Input: part model. Units: mm. Frame: model coordinates. Face numbers are marked on the shaded views. A direction names the side the tool comes from. Give positions to 0.01 mm unless a question says otherwise; leave off trailing zeros. Write each loop counter-clockwise with the first axis right and the second up, starting at its lowest first coordinate (ties: lowest second). Pieces come first, ordered by that corner, then holes. Notation, with made-up numbers: M -34,-40 L -14,-40 A15 cw -14,-27 Z; hole C 12.25,34.25 d7. An arc over 180 degrees is marked long. Use CSV: the item, a comma, the result in double quotes. Start each with the question number.
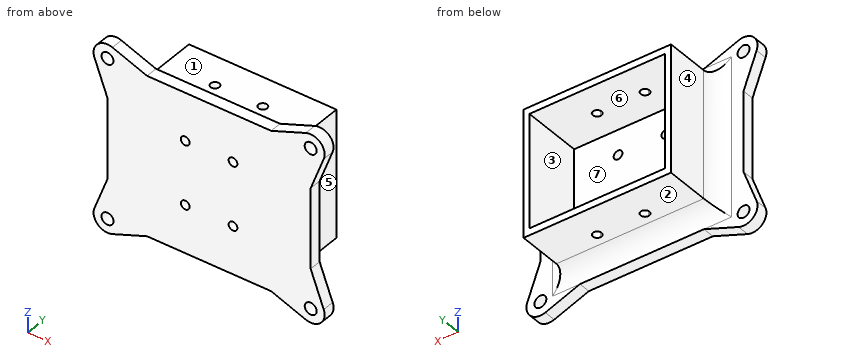
from build123d import *

# Parameters (mm, degrees)
SKETCH1_R               = 1.5
BOSS_EXTRUDE2_DEPTH     = 3
SKETCH2_W               = 37
SKETCH2_H               = 32
SKETCH2_W_2             = 34.05
SKETCH2_H_2             = 28.55
BOSS_EXTRUDE3_DEPTH     = 15
CUT_EXTRUDE1_DEPTH      = 40
CUT_EXTRUDE1_DEPTH_BACK = 11
SKETCH2_4_R             = 1.1
CUT_EXTRUDE2_DEPTH      = 11
FILLET1_R               = 4


with BuildPart() as part:
    # Sketch1 → Boss-Extrude2 (new body)
    with BuildSketch(Plane(origin=(0, 0, 0), x_dir=(1, 0, 0), z_dir=(0, 1, 0))):
        with BuildLine():
            Line((-24.266499455, 23.2754353), (-15.568913997, 20))
            Line((-15.568913997, 20), (15.568913997, 20))
            Line((15.568913997, 20), (24.266499455, 23.2754353))
            ThreePointArc((24.266499455, 23.2754353), (27.974873734, 22.474873734), (28.7754353, 18.766499455))
            Line((28.7754353, 18.766499455), (25.5, 10.068913997))
            Line((25.5, 10.068913997), (25.5, -10.068913997))
            Line((25.5, -10.068913997), (28.7754353, -18.766499455))
            ThreePointArc((28.7754353, -18.766499455), (27.974873734, -22.474873734), (24.266499455, -23.2754353))
            Line((24.266499455, -23.2754353), (15.568913997, -20))
            Line((15.568913997, -20), (-15.568913997, -20))
            Line((-15.568913997, -20), (-24.266499455, -23.2754353))
            ThreePointArc((-24.266499455, -23.2754353), (-27.974873734, -22.474873734), (-28.7754353, -18.766499455))
            Line((-28.7754353, -18.766499455), (-25.5, -10.068913997))
            Line((-25.5, -10.068913997), (-25.5, 10.068913997))
            Line((-25.5, 10.068913997), (-28.7754353, 18.766499455))
            ThreePointArc((-28.7754353, 18.766499455), (-27.974873734, 22.474873734), (-24.266499455, 23.2754353))
        make_face()
        with Locations(Location((-25.5, 20, 0), (0, 0, 270))):
            Circle(SKETCH1_R, mode=Mode.SUBTRACT)
        with Locations(Location((25.5, 20, 0), (0, 0, 270))):
            Circle(SKETCH1_R, mode=Mode.SUBTRACT)
        with Locations(Location((25.5, -20, 0), (0, 0, 270))):
            Circle(SKETCH1_R, mode=Mode.SUBTRACT)
        with Locations(Location((-25.5, -20, 0), (0, 0, 270))):
            Circle(SKETCH1_R, mode=Mode.SUBTRACT)
    extrude(amount=BOSS_EXTRUDE2_DEPTH)

    # Sketch2 → Boss-Extrude3 (add)
    with BuildSketch(Plane(origin=(0, 3, 0), x_dir=(1, 0, 0), z_dir=(0, 1, 0))):
        Rectangle(SKETCH2_W, SKETCH2_H)
        Rectangle(SKETCH2_W_2, SKETCH2_H_2, mode=Mode.SUBTRACT)
    extrude(amount=BOSS_EXTRUDE3_DEPTH)

    # Sketch3 → Cut-Extrude1 (cut, two sides: drawn at the far end of the back side and taken through both)
    with BuildSketch(Plane.XY.offset(-14.275).offset(-CUT_EXTRUDE1_DEPTH_BACK)):
        with BuildLine():
            ThreePointArc((-4.9, 10), (-6.777817459, 10.777817459), (-6, 8.9))
            Line((-6, 8.9), (-6, 10))
            Line((-6, 10), (-4.9, 10))
        make_face()
        with BuildLine():
            Line((-6, 10), (-6, 8.9))
            ThreePointArc((-6, 8.9), (-5.222182541, 9.222182541), (-4.9, 10))
            Line((-4.9, 10), (-6, 10))
        make_face()
        with BuildLine():
            ThreePointArc((4.9, 10), (5.222182541, 9.222182541), (6, 8.9))
            Line((6, 8.9), (6, 10))
            Line((6, 10), (4.9, 10))
        make_face()
        with BuildLine():
            Line((6, 10), (6, 8.9))
            ThreePointArc((6, 8.9), (6.777817459, 9.222182541), (7.1, 10))
            ThreePointArc((7.1, 10), (6, 11.1), (4.9, 10))
            Line((4.9, 10), (6, 10))
        make_face()
    extrude(amount=CUT_EXTRUDE1_DEPTH + CUT_EXTRUDE1_DEPTH_BACK, mode=Mode.SUBTRACT)

    # Sketch2<4> → Cut-Extrude2 (cut)
    with BuildSketch(Plane(origin=(0, 3, 0), x_dir=(1, 0, 0), z_dir=(0, 1, 0))):
        with Locations(Location((-6, 8, 0), (0, 0, 270))):
            Circle(SKETCH2_4_R)
        with Locations(Location((6, 8, 0), (0, 0, 270))):
            Circle(SKETCH2_4_R)
        with Locations(Location((6, -8, 0), (0, 0, 270))):
            Circle(SKETCH2_4_R)
        with Locations(Location((-6, -8, 0), (0, 0, 270))):
            Circle(SKETCH2_4_R)
    extrude(amount=-CUT_EXTRUDE2_DEPTH, mode=Mode.SUBTRACT)

    # Fillet1
    fillet1_edges = [part.edges().sort_by_distance(p)[0] for p in [
        (-18.5, 3, 0),
        (0, 3, 16),
        (18.5, 3, 0),
        (0, 3, -16),
    ]]
    fillet(fillet1_edges, radius=FILLET1_R - 0.0001)  # a hair under: the kernel refuses the full size


solid = part.part
Q1. Set-up query: the marked faces 1, 2 and 3. Return all of +Z, -Z, +X, -X, +Y, -Y with unobstructed straight access to the full face (end or side cutting, diameter ignored); none if empty.
Q2. Section B-B, the plane z = -2.5. Return the cut outline in (x, y) (3 decimals), and give its area (3 significant figures).
Q3. Section A-A, the plane y = 11.75. Return the cut outline in (x, z) (3 decimals), and give its area (3 significant figures).
Q4. Pull-direction query (X, two-part tool) for the marked faces 4, 5, 6 and 7; classes: released by +X, released by -X, zero draft, split by the parting line, or undercut.
Q5. Material intervals for L1, parallel to X at y = 10, z = -15.3; L2, parallel to X at y = 1.1, z = -8; L3, parallel to Z at x = -13.5, y = 10.75 (3 decimals), sorted ascending. Write a range as [from, to].
Q6. Section C-C, the plane y = 2. Give the number of separate pieces and of enclosed holes in the cut face, and give its area (3 significant figures).
Q7. First-contact query: pin 1 Ø0.9 at (x, y) = (7, 1) entering from -Z; pin 2 Ø3 at (x, y) = (-13, 7.5) entering from -Z; pin 3 Ø6 at (y, z) = (14.5, 3.5) entering from +X; pin 4 Ø2 at (x, z) = (6, -8) entering from -Y. Flat tips, straight axial feed; report the tip coordinate or a pass-through.
Check result:
1,face 1,"+Z, +X, -X, +Y"
1,face 2,"-Z, +X, -X, +Y"
1,face 3,"+Y"
2,outline,"M -25.5,0 L 25.5,0 L 25.5,3 L 22.5,3 A4 cw 18.5,7 L 18.5,18 L 17.025,18 L 17.025,3 L -17.025,3 L -17.025,18 L -18.5,18 L -18.5,7 A4 cw -22.5,3 L -25.5,3 Z"
2,area,"204 mm²"
3,outline,"M -18.5,-16 L 18.5,-16 L 18.5,16 L -18.5,16 Z; hole M -17.025,-14.275 L 17.025,-14.275 L 17.025,14.275 L -17.025,14.275 Z"
3,area,"212 mm²"
4,face 4,"released by -X"
4,face 5,"released by +X"
4,face 6,"undercut"
4,face 7,"undercut"
5,L1,"x = [-18.5, -7.1], [-4.9, 4.9], [7.1, 18.5]"
5,L2,"x = [-25.5, -7.1], [-4.9, 4.9], [7.1, 25.5]"
5,L3,"z = [-16, -14.275], [14.275, 16]"
6,separate pieces,"1"
6,enclosed holes,"8"
6,area,"2,180 mm²"
7,pin 1,"stops at z = -20"
7,pin 2,"stops at z = -16.13"
7,pin 3,"stops at x = 18.5"
7,pin 4,"passes through"
